Check sheet for the modelled part. Datum: model origin and axes. Units: mm. Face numbers are marked on the shaded views. A direction names the side the tool comes from. Round coordinates to 2 decimals unless told otherwise and drop trailing zeros. Order: outer loops, then holes, each group sorted by start corner. A loop starts at its lowest first (then second) coordinate and runs counter-clockwise, first axis right, second up.
Autodesk Inventor part; units mm, degrees
ref_plane "YZ Plane" through (0, 0, 0) normal (1, 0, 0) x (0, 1, 0)
ref_plane "XZ Plane" through (0, 0, 0) normal (0, 1, 0) x (-1, 0, 0)
ref_plane "XY Plane" through (0, 0, 0) normal (0, 0, 1) x (1, 0, 0)
sketch "Sketch1" plane through (0, 0, 0) normal (0, 1, 0) x (-1, 0, 0)
  line L0 (0, 88.9) -> (0, -88.9) construction
  line L1 (25.4, 63.5) -> (25.4, -63.5)
  line L2 (-25.4, -63.5) -> (-25.4, 63.5)
  arc A0 (25.4, 63.5) -> (-25.4, 63.5) centre (0, 63.5) ccw
  arc A1 (-25.4, -63.5) -> (25.4, -63.5) centre (0, -63.5) ccw
  circle A2 centre (0, 63.5) radius 6.35
  circle A3 centre (0, -63.5) radius 6.35
  point P0 (0, 0)
  point P1 (0, 0)
  dimension "d0" = 127
  dimension "d1" = 12.7
  dimension "d2" = 12.7
  dimension "d3" = 25.4
extrude "BASE" add sketch "Sketch1" along normal blind 12.7
sketch "Sketch2" plane through (0, 0, 0) normal (1, 0, 0) x (0, 1, 0)
  arc A0 (0, -44.45) -> (0, 44.45) centre (0, 0) ccw
  arc A1 (0, -31.75) -> (0, 31.75) centre (0, 0) ccw
  line L0 (0, -63.5) -> (0, 63.5)
  line L1 (0, 31.75) -> (15.875, 31.75)
  line L2 (15.875, 31.75) -> (15.875, -31.75)
  line L3 (15.875, -31.75) -> (0, -31.75)
  line L4 (0, -31.75) -> (0, 31.75)
  line L5 (0, 63.5) -> (0, -63.5)
  point P0 (7.9375, -31.75)
  point P1 (0, 0)
  point P2 (15.875, -27.4963)
  point P3 (15.875, 27.4963)
  point P4 (0, -31.75)
  dimension "d7" = 44.45
  dimension "d8" = 31.75
  dimension "d16" = 63.5
  dimension "d17" = 31.75
  dimension "d18" = 15.875
extrude "REMOVED CENTER OF BASE" cut sketch "Sketch2" along normal through all both and the other way through all
extrude "ARCH" add sketch "Sketch2" along normal mid plane 63.5
sketch "Sketch3" plane through (0, 0, 0) normal (0, 1, 0) x (-1, 0, 0)
  circle A0 centre (0, 0) radius 3.175
  dimension "d13" = 6.35
extrude "TOPHOLE" cut sketch "Sketch3" along normal through all
sketch "Sketch5" plane through (31.75, 0, 0) normal (1, 0, 0) x (0, 0, -1)
  line L0 (-44.45, 0) -> (44.45, 0)
  circle A0 centre (0, 0) radius 31.75
  point P0 (-31.75, 0)
  dimension "d26" = 31.75
extrude "CIRCULAR" [suppressed]
sketch "Sketch6" plane through (31.75, 0, 0) normal (1, 0, 0) x (0, 0, -1)
  line L0 (-25.4, 25.4) -> (25.4, 25.4)
  line L1 (25.4, 25.4) -> (25.4, 0)
  line L2 (25.4, 0) -> (-25.4, 0)
  line L3 (-25.4, 0) -> (-25.4, 25.4)
  point P0 (0, 0)
  point P1 (0, 0)
  point P2 (0, 0)
  dimension "d23" = 50.8
  dimension "d24" = 25.4
  dimension "d25" = 25.4
extrude "SQUARE" cut sketch "Sketch6" against normal through all
equation "\"d2\" = d1"
equation "\"d11\" = d16"
properties part number "ANS7S-TUT-BK" material "Brass, Soft Yellow, Welded"
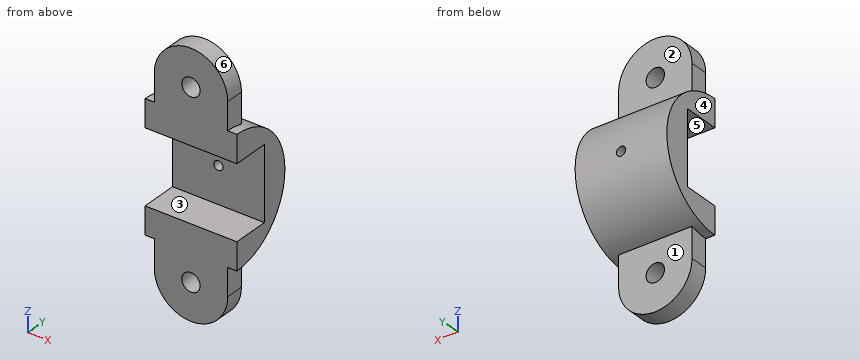
Item 1: Scan lines: line 1 along Z through (x, y) = (0, 10); line 2 along X through (y, z) = (7, -63); line 3 along X through (y, z) = (35.75, 0) (3 decimals). Record each from-to range of solid material in increasing order.
Answer:
line 1: z = -88.9 to -69.85, -57.15 to -25.4, 25.4 to 57.15, 69.85 to 88.9
line 2: x = -25.4 to -6.33, 6.33 to 25.4
line 3: x = -31.75 to -3.175, 3.175 to 31.75
Item 2: Access from +Z, -Z, +X, -X, +Y, -Y to the whole of each face (thin tool, end or side, straight path). Record for the marked faces 1, 2 and 3.
Answer:
face 1: -Z, +X, -X, +Y
face 2: +Z, +X, -X, +Y
face 3: +X, -X, -Y
Item 3: Sectioned sample at C-C (x = 0). Record the cut outline in (y, z) (3 decimals).
Answer:
outline: (0, -88.9) - (12.7, -88.9) - (12.7, -69.85) - (0, -69.85) - close; (0, -57.15) - (12.7, -57.15) - (12.7, -42.597) arc R44.45 ccw to (44.336, -3.175) - (25.4, -3.175) - (25.4, -25.4) - (0, -25.4) - close; (0, 25.4) - (25.4, 25.4) - (25.4, 3.175) - (44.336, 3.175) arc R44.45 ccw to (12.7, 42.597) - (12.7, 57.15) - (0, 57.15) - close; (0, 69.85) - (12.7, 69.85) - (12.7, 88.9) - (0, 88.9) - close
Item 4: Release check for a two-part mould opening along Z. For the marked faces 4, 5 and 6 record: released by +Z, released by -Z, zero draft, split by the parting line, or undercut.
Answer:
face 4: zero draft
face 5: undercut
face 6: released by +Z
Item 5: Sectioned sample at B-B (y = 10.5). Record the cut outline in (x, z).
Answer:
outline: (-31.75, -43.19) - (-25.4, -43.19) - (-25.4, -63.5) arc R25.4 ccw to (25.4, -63.5) - (25.4, -43.19) - (31.75, -43.19) - (31.75, -25.4) - (-31.75, -25.4) - close; (-31.75, 25.4) - (31.75, 25.4) - (31.75, 43.19) - (25.4, 43.19) - (25.4, 63.5) arc R25.4 ccw to (-25.4, 63.5) - (-25.4, 43.19) - (-31.75, 43.19) - close; hole circle Ø12.7 at (0, -63.5); hole circle Ø12.7 at (0, 63.5)
Item 6: Sectioned sample at A-A (z = 0). Record the cut outline in (x, y) (3 decimals).
Answer:
outline: (-31.75, 25.4) - (-3.175, 25.4) - (-3.175, 44.45) - (-31.75, 44.45) - close; (3.175, 25.4) - (31.75, 25.4) - (31.75, 44.45) - (3.175, 44.45) - close
Item 7: Sectioned sample at D-D (y = 22.5). Record the cut outline in (x, z).
Answer:
outline: (-31.75, -38.33) - (31.75, -38.33) - (31.75, -25.4) - (-31.75, -25.4) - close; (-31.75, 25.4) - (31.75, 25.4) - (31.75, 38.33) - (-31.75, 38.33) - close
Item 8: Go/stop test with flat-tipped pins: P1, Ø20.5, axis at x = 0, z = 63.5, coming from the +Y side; P2, Ø11.5, axis at x = 0, z = -63.5, coming from the -Y side; P3, Ø2, axis at x = 1.5, z = 18, coming from the +Y side; P4, Ø10, axis at y = 6, z = -53, coming from the -X side. Record where each tip stops, or that it passes through.
Answer:
P1: stops at y = 12.7
P2: passes through
P3: stops at y = 41.07
P4: stops at x = -25.4
